from build123d import *

# Parameters (mm, degrees)
F0_W     = 100
F0_H     = 100
F1_DEPTH = 90
F2_W     = 64.8323260248
F2_H     = 70.6382095814
F3_DEPTH = 50
F4_W     = 65.3021298349
F4_H     = 31.1890766025
F5_DEPTH = 25
F6_DEPTH = 50
F8_R     = 1


# Not quite as in the source:
# - a feature of the source that left no trace in its solid (it failed there, or was rolled back) is left out


with BuildPart() as f1:
    # F0 (on Top) → F1 (new body)
    with BuildSketch(Plane.XY):
        Rectangle(F0_W, F0_H)
    extrude(amount=F1_DEPTH)

    # F2 (on Front) → F3 (cut)
    with BuildSketch(Plane.XZ):
        with Locations((-0.7257331163, 55.6396842003)):
            Rectangle(F2_W, F2_H)
    extrude(amount=F3_DEPTH, mode=Mode.SUBTRACT)

    # F4 (on Top) → F5 (join)
    with BuildSketch(Plane.XY):
        with Locations((-0.2436619252, 15.5945383012)):
            Rectangle(F4_W, F4_H)
    extrude(amount=F5_DEPTH)

    # F4 (on Top) → F6 (join)
    with BuildSketch(Plane.XY):
        with Locations((-0.2436619252, 15.5945383012)):
            Rectangle(F4_W, F4_H)
    extrude(amount=F6_DEPTH)

    # F8
    f8_edges = [f1.edges().sort_by_distance(p)[0] for p in [
        (-33.141896, -25, 90),
        (31.69043, -25, 90),
        (40.845215, -50, 90),
        (50, 0, 90),
        (0, 50, 90),
        (-50, 0, 90),
        (-50, 50, 45),
        (-50, 0, 0),
        (-41.570948, -50, 90),
        (-33.141896, -50, 55.16029),
        (0, -50, 0),
        (-0.725733, -50, 20.320579),
        (31.69043, -25, 20.320579),
        (31.69043, -50, 55.16029),
        (50, -50, 45),
        (-0.725733, 0, 20.320579),
        (-33.141896, -25, 20.320579),
        (-33.141896, 0, 55.16029),
        (-50, -50, 45),
        (50, 50, 45),
        (50, 0, 0),
        (0, 50, 0),
        (-0.725733, 0, 90),
    ]]
    fillet(f8_edges, radius=F8_R)


solid = f1.part
Geometry: final body of the model. Coordinates: model frame, mm. A direction names the side the tool comes from. Give positions to 0.01 mm unless a question says otherwise; leave off trailing zeros. Write each loop counter-clockwise with the first axis right and the second up, starting at its lowest first coordinate (ties: lowest second). Pieces come first, ordered by that corner, then holes. Notation, with made-up numbers: (85.5, 21.25) - (112.5, 21.25) arc R17 cw to (112.5, 29.25) - close; hole circle Ø2 at (60, -26.5). An arc over 180 degrees is marked (long way). Return JSON: item names as keys, results as strings. Group by question number.
1) Set-up query: faces 1 (the flat face through (-1, -50, 15)), 2 (the flat face through (-1, 0, 56)). Return all of +Z, -Z, +X, -X, +Y, -Y with unobstructed straight access to the full face (end or side cutting, diameter ignored); none if empty.
2) Mould query, pull axis X, two halves, no side actions, for faces 3 (the flat face through (-1, 50, 44)), 4 (the flat face through (-33.142, -25, 55)), 5 (the flat face through (-50, -1, 44)), 6 (the flat face through (50, -1, 44)). Classes: released by +X, released by -X, zero draft, split by the parting line, or undercut.
3) Section B-B on x = 8. Return the cut outline in (y, z).
4) First-contact query: P1, Ø14.5, axis at x = -5.5, y = -25.5, coming from the +Z side; P2, Ø19, axis at x = 9, z = 41.5, coming from the -Y side. Flat tips, straight axial feed; report the tip coordinate or a pass-through.
5) Section A-A on z = 54. Return the cut outline in (x, y), plus the area to 3 significant figures.
6) Section C-C on y = -13. Return the cut outline in (x, z), plus the area to 3 significant figures.
7) Line query: line 1 (X direction, y = -19, z = 47.5); line 2 (Y direction, x = -34, z = 35); line 3 (Y direction, x = 15, z = 51.5). Output: solid intervals per line, ascending.
Filled in:
{
 "1": {"face 1": "+Z, -Z, +X, -X, -Y", "face 2": "+Z, -Y"},
 "2": {"face 3": "zero draft", "face 4": "undercut", "face 5": "released by -X", "face 6": "released by +X"},
 "3": {"outline": "(-50, 1) arc R1 ccw to (-49, 0) - (49, 0) arc R1 ccw to (50, 1) - (50, 89) arc R1 ccw to (49, 90) - (1, 90) arc R1 ccw to (0, 89) - (0, 21.32) arc R1 cw to (-1, 20.32) - (-49, 20.32) arc R1 ccw to (-50, 19.32) - close"},
 "4": {"P1": "stops at z = 20.32", "P2": "stops at y = 0"},
 "5": {"outline": "(-50, -49) arc R1 ccw to (-49, -50) - (-34.14, -50) arc R1 ccw to (-33.14, -49) - (-33.14, -1) arc R1 cw to (-32.14, 0) - (31.69, 0) - (31.69, -49) arc R1 ccw to (32.69, -50) - (49, -50) arc R1 ccw to (50, -49) - (50, 49) arc R1 ccw to (49, 50) - (-49, 50) arc R1 ccw to (-50, 49) - close", "area": "6,760 mm^2"},
 "6": {"outline": "(-50, 1) arc R1 ccw to (-49, 0) - (49, 0) arc R1 ccw to (50, 1) - (50, 89) arc R1 ccw to (49, 90) - (32.69, 90) arc R1 ccw to (31.69, 89) - (31.69, 21.32) arc R1 cw to (30.69, 20.32) - (-32.14, 20.32) arc R1 cw to (-33.14, 21.32) - (-33.14, 89) arc R1 ccw to (-34.14, 90) - (-49, 90) arc R1 ccw to (-50, 89) - close", "area": "4,480 mm^2"},
 "7": {"line 1": "x = -50 to -33.14, 31.69 to 50", "line 2": "y = -49.99 to 50", "line 3": "y = 0 to 50"}
}
